Job drawing, mm, ordinate dimensions from the low corner. One solid piece. Give positions to 0.01 mm unless a question says otherwise; leave off trailing zeros. Order: outer loops, then holes, each group sorted by start corner. A loop starts at its lowest first (then second) coordinate and runs counter-clockwise, first axis right, second up. Notation, with made-up numbers: M 78,63.5 L 127,63.5 A14 ccw 127,85.5 Z; hole C 16.5,56 d7. An arc over 180 degrees is marked long. One line per item, written item: value. Start each with the question number.
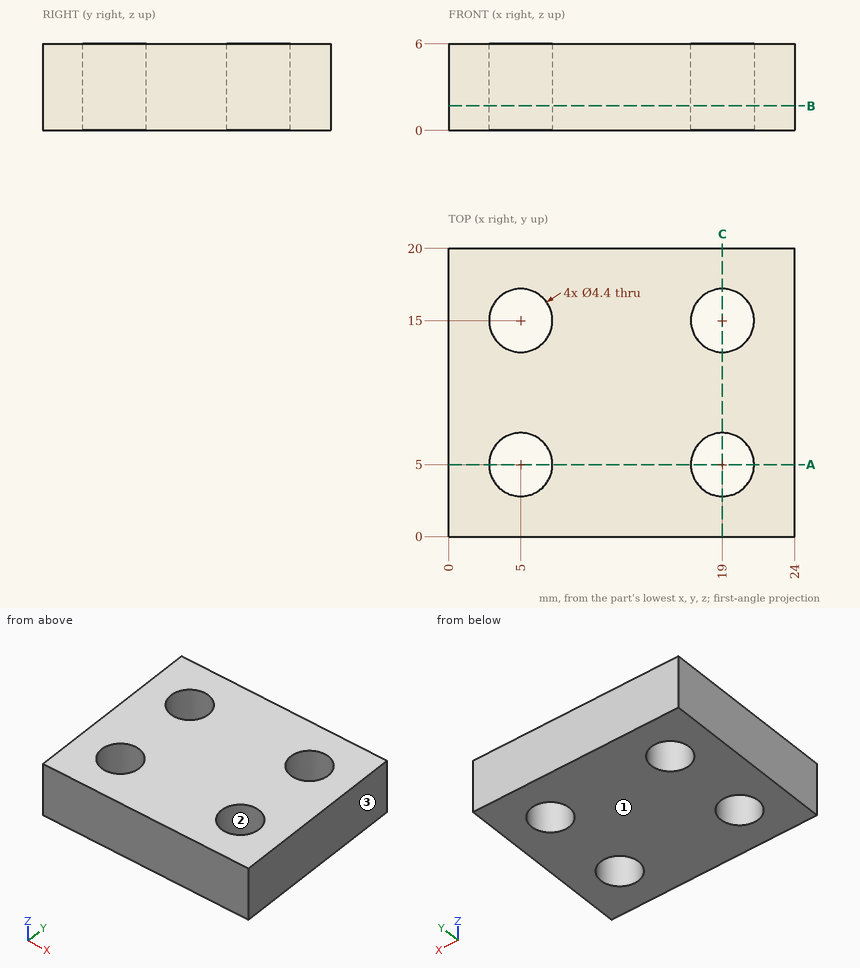
1) Drop flat-ended pins along their axis: P1, Ø7, axis at x = 5, y = 5, coming from the -Z side; P2, Ø3.5, axis at x = 19, y = 15, coming from the +Z side. Give the stop position or say it passes through.
2) Slice it at A-A (y = 5). List the corners of the cut face in (x, z).
3) Drill centre lines: line 1 (Y direction, x = 5, z = 4.8); line 2 (X direction, y = 6, z = 1.8); line 3 (X direction, y = 16.75, z = 5). Where is each one in solid material? Low to high.
4) Slice it at B-B (z = 1.7). List the corners of the cut face in (x, y).
5) Slice it at C-C (x = 19). List the corners of the cut face in (y, z), plus the area to 3 significant figures.
6) Pull direction X, two halves, no side cores. Call the marked faces 1, 2 and 3: pulls with the +X half, pulls with the -X half, needs draft (parallel to the pull), parting line crosses it, or undercut.
Results list:
1. P1: stops at z = 0
1. P2: passes through
2. outline: M 0,0 L 2.8,0 L 2.8,6 L 0,6 Z; M 7.2,0 L 16.8,0 L 16.8,6 L 7.2,6 Z; M 21.2,0 L 24,0 L 24,6 L 21.2,6 Z
3. line 1: y = 0 to 2.8, 7.2 to 12.8, 17.2 to 20
3. line 2: x = 0 to 3.04, 6.96 to 17.04, 20.96 to 24
3. line 3: x = 0 to 3.67, 6.33 to 17.67, 20.33 to 24
4. outline: M 0,0 L 24,0 L 24,20 L 0,20 Z; hole C 5,5 d4.4; hole C 5,15 d4.4; hole C 19,5 d4.4; hole C 19,15 d4.4
5. outline: M 0,0 L 2.8,0 L 2.8,6 L 0,6 Z; M 7.2,0 L 12.8,0 L 12.8,6 L 7.2,6 Z; M 17.2,0 L 20,0 L 20,6 L 17.2,6 Z
5. area: 67.2 mm²
6. face 1: needs draft
6. face 2: undercut
6. face 3: pulls with the +X half
